Here's how the part is built. I have some questions about the finished solid (model axes, mm). A direction names the side the tool comes from. Round coordinates to 2 decimals unless told otherwise and drop trailing zeros. Order: outer loops, then holes, each group sorted by start corner. A loop starts at its lowest first (then second) coordinate and runs counter-clockwise, first axis right, second up. Notation, with made-up numbers: (19, 0.5) -> (62, 0.5) arc R5 ccw to (62, 7.5) -> close; hole circle Ø8 at (89, 75). An arc over 180 degrees is marked (long way). One line per item, written item: value.
```python
from build123d import *

# Parameters (mm, degrees)
SKETCH1_W           = 47.625
SKETCH1_H           = 47.625
BOSS_EXTRUDE1_DEPTH = 2
BOSS_EXTRUDE2_DEPTH = 4
SKETCH4_R           = 1.5
CUT_EXTRUDE2_DEPTH  = 69.068210275
SKETCH5_W           = 47.625
SKETCH5_H           = 47.625
SKETCH5_W_2         = 44.625
SKETCH5_H_2         = 44.625
BOSS_EXTRUDE3_DEPTH = 10
SKETCH6_W           = 8
SKETCH6_H           = 7
CUT_EXTRUDE3_DEPTH  = 2


with BuildPart() as part:
    # Sketch1 → Boss-Extrude1 (new body)
    with BuildSketch(Plane(origin=(0, 0, 0), x_dir=(1, 0, 0), z_dir=(0, 1, 0))):
        with Locations((23.8125, 23.8125)):
            Rectangle(SKETCH1_W, SKETCH1_H)
    extrude(amount=BOSS_EXTRUDE1_DEPTH)

    # Sketch2 → Boss-Extrude2 (add)
    with BuildSketch(Plane.XZ):
        Polygon((15.680772016, -28.408694078), (28.408694078, -15.680772016), (31.944227984, -19.216305922), (19.216305922, -31.944227984), align=None)
    extrude(amount=BOSS_EXTRUDE2_DEPTH)

    # Sketch4 → Cut-Extrude2 (cut, through all)
    with BuildSketch(Plane(origin=(6.363961031, 0, 6.363961031), x_dir=(0.7071067811865475, 0, -0.7071067811865477), z_dir=(0.7071067811865477, 0, 0.7071067811865475))):
        with Locations(Location((33.675960454, -1.5, 0), (0, 0, 90))):
            Circle(SKETCH4_R)
    extrude(amount=-CUT_EXTRUDE2_DEPTH, mode=Mode.SUBTRACT)

    # Sketch5 → Boss-Extrude3 (add)
    with BuildSketch(Plane.XZ):
        with Locations((23.8125, -23.8125)):
            Rectangle(SKETCH5_W, SKETCH5_H)
        with Locations((23.8125, -23.8125)):
            Rectangle(SKETCH5_W_2, SKETCH5_H_2, mode=Mode.SUBTRACT)
    extrude(amount=BOSS_EXTRUDE3_DEPTH)

    # Sketch6 → Cut-Extrude3 (cut)
    with BuildSketch(Plane.XY):
        with Locations((23.8125, -6.5)):
            Rectangle(SKETCH6_W, SKETCH6_H)
    extrude(amount=-CUT_EXTRUDE3_DEPTH, mode=Mode.SUBTRACT)


solid = part.part
```
Q1. I want a section at B-B on y = -1.5. Write out the boundary of the cut face in (x, z) (3 decimals), then the cut area to 3 significant figures.
Answers:
outline: (0, -47.625) -> (47.625, -47.625) -> (47.625, 0) -> (0, 0) -> close; (15.681, -28.409) -> (16.388, -29.116) -> (29.116, -16.388) -> (28.409, -15.681) -> close; (18.509, -31.237) -> (19.216, -31.944) -> (31.944, -19.216) -> (31.237, -18.509) -> close; hole (1.5, -46.125) -> (46.125, -46.125) -> (46.125, -1.5) -> (1.5, -1.5) -> close
area: 313 mm2
Q2. I need wall thicknesses on line 1 along X through (y, z) = (-9.5, -23.5) (3 decimals); line 2 along Z through (x, y) = (15.5, -6.25) (3 decimals); line 3 along Z through (x, y) = (23.5, -2.25) (3 decimals). Which ranges of each line are inside material? Lowest first, please.
Answers:
line 1: 0 to 1.5, 46.125 to 47.625
line 2: -47.625 to -46.125, -1.5 to 0
line 3: -47.625 to -46.125, -27.661 to -25.962, -22.288 to -20.589, -1.5 to 0
Q3. For P1, Ø8, axis at x = 13.5, z = -15.5, coming from the -Y side; P2, Ø0.8, axis at x = 23, z = -1, coming from the -Y side, each with a flat end and sliding along its axis, tell me the tip position at first contact or that it passes through.
Answers:
P1: y = 0
P2: y = -3
Q4. Which directions (+Z, -Z, +X, -X, +Y, -Y) give clear straight access to the entire face, cutting with the end or side of a thin tool? Please do faces 1 (the face through (19.812, -7, -1)), 2 (the face through (21.96, -1.97, -22.13)), 3 (the face through (24, -10, -47)).
Answers:
face 1: +Z, -Y
face 2: -Y
face 3: +Z, -Z, +X, -X, -Y
Q5. If we mould it in two halves opening along X, with no side actions, what happens to faces 4 (the face through (47.625, -4, -24)), 5 (the face through (24, -3, -1)), 6 (the face through (23, -4, -47.625))? For each: pulls with the +X half, pulls with the -X half, needs draft (parallel to the pull), parting line crosses it, or undercut.
Answers:
face 4: pulls with the +X half
face 5: undercut
face 6: needs draft
Q6. I want a section at D-D on y = -7.5. Write out the boundary of the cut face in (x, z) (1 decimal), then the cut area to 3 significant figures.
Answers:
outline: (0, -47.6) -> (47.6, -47.6) -> (47.6, 0) -> (27.8, 0) -> (27.8, -1.5) -> (46.1, -1.5) -> (46.1, -46.1) -> (1.5, -46.1) -> (1.5, -1.5) -> (19.8, -1.5) -> (19.8, 0) -> (0, 0) -> close
area: 265 mm2
Q7. I want a section at C-C on x = 12. Write out the boundary of the cut face in (y, z) (3 decimals), then the cut area to 3 significant figures.
Answers:
outline: (-10, -47.625) -> (2, -47.625) -> (2, 0) -> (-10, 0) -> (-10, -1.5) -> (0, -1.5) -> (0, -46.125) -> (-10, -46.125) -> close
area: 125 mm2
Q8. I want a section at A-A on z = -11. Write out the boundary of the cut face in (x, y) (3 decimals), then the cut area to 3 significant figures.
Answers:
outline: (0, -10) -> (1.5, -10) -> (1.5, 0) -> (46.125, 0) -> (46.125, -10) -> (47.625, -10) -> (47.625, 2) -> (0, 2) -> close
area: 125 mm2
